Design review of the part built by this model. Coordinates are the model's own, in mm. A direction names the side the tool comes from. Coordinates: 2 decimals unless noted, no trailing zeros. Loops run counter-clockwise (first coordinate to the right, second up) from the corner with the lowest first, then second, coordinate; pieces in that order, holes last. Notation, with made-up numbers: (53.25, -16.75) - (89.25, -16.75) arc R7 ccw to (89.25, -12.75) - close; hole circle Ø5 at (61.25, 13). An arc over 180 degrees is marked (long way). Answer in a Markdown table with one row per item. Add a question column.
(1) Clearance check with flat-ended pins moving along their axes: pin 1 (1 mm diameter, centred on x = 10, y = 19.5, fed in from +Z); pin 2 (9 mm diameter, centred on y = 19.5, z = -10, fed in from -X); pin 3 (7.5 mm diameter, centred on x = 11, z = -7, fed in from +Y). State where each tip first meets the part, or that it passes through.
(2) We need section C-C, the plane y = 12.75. Write out the cut boundary in (x, z), plus the area to 3 significant figures.
(3) To check wall thickness, follow L1, parallel to X at y = 15, z = -11; L2, parallel to Y at x = 15, z = -1.5; L3, parallel to Z at x = 17.25, y = 13.25. State the ranges of each line that lie inside material, in increasing order. Write a range as [from, to].
(4) For faces 1 (the face through (20, 10, -16)), 2 (the face through (2.54, 11, -14)), list the 3-axis set-ups (+Z, -Z, +X, -X, +Y, -Y) from which the entire face can be reached by the end or side of a thin tool; tool diameter is ignored.
(5) The part is to be moulded in two halves that separate along X. For faces 3 (the face through (10, 6.35, -7)), 4 (the face through (12, 14, -19.05)), 5 (the face through (0, 9, -16)), 6 (the face through (10, 13, -25.4)), say which applies: released by +X, released by -X, zero draft, split by the parting line, or undercut.
(6) We need section B-B, the plane z = -20. Write out the cut boundary in (x, y) (3 decimals).
(7) We need section A-A, the plane y = 2. Write out the cut boundary in (x, z) (3 decimals).
(8) We need section D-D, the plane x = 10.25. Write out the cut boundary in (y, z), plus the area to 3 significant figures.
from build123d import *

# Parameters (mm, degrees)
BOSS_EXTRUDE1_DEPTH = 20
CUT_EXTRUDE1_DEPTH  = 20
CUT_EXTRUDE2_DEPTH  = 20
FILLET1_R           = 6.35
BOSS_EXTRUDE2_DEPTH = 19.05
CUT_EXTRUDE3_DEPTH  = 20.05
CUT_EXTRUDE4_DEPTH  = 21


with BuildPart() as part:
    # Sketch1 → Boss-Extrude1 (new body)
    with BuildSketch(Plane(origin=(0, 0, 0), x_dir=(0, 0, -1), z_dir=(1, 0, 0))):
        Polygon((0, 0), (0, 6.35), (19.05, 6.35), (19.05, 25.4), (25.4, 25.4), (25.4, 0), align=None)
    extrude(amount=BOSS_EXTRUDE1_DEPTH)

    # Sketch2 → Cut-Extrude1 (cut)
    with BuildSketch(Plane(origin=(0, 6.35, 0), x_dir=(1, 0, 0), z_dir=(0, 1, 0))):
        with BuildLine():
            ThreePointArc((8.37078656, 11.076825802), (7.750000055, 9.525), (8.37078656, 7.973174198))
            Line((8.37078656, 7.973174198), (10, 9.525))
            Line((10, 9.525), (8.37078656, 11.076825802))
        make_face()
        with BuildLine():
            Line((10, 9.525), (8.37078656, 7.973174198))
            ThreePointArc((8.37078656, 7.973174198), (10, 7.275000055), (11.62921344, 7.973174198))
            Line((11.62921344, 7.973174198), (10, 9.525))
        make_face()
        with BuildLine():
            Line((8.37078656, 11.076825802), (10, 9.525))
            Line((10, 9.525), (11.62921344, 11.076825802))
            ThreePointArc((11.62921344, 11.076825802), (10, 11.774999945), (8.37078656, 11.076825802))
        make_face()
        with BuildLine():
            Line((11.62921344, 11.076825802), (10, 9.525))
            Line((10, 9.525), (11.62921344, 7.973174198))
            ThreePointArc((11.62921344, 7.973174198), (12.089046422, 8.689305797), (12.249999945, 9.525))
            ThreePointArc((12.249999945, 9.525), (12.089046422, 10.360694203), (11.62921344, 11.076825802))
        make_face()
    extrude(amount=-CUT_EXTRUDE1_DEPTH, mode=Mode.SUBTRACT)

    # Sketch3 → Cut-Extrude2 (cut)
    with BuildSketch(Plane.XY.offset(-19.05)):
        with BuildLine():
            ThreePointArc((8.37078652, 17.42682584), (7.75, 15.875), (8.37078652, 14.32317416))
            Line((8.37078652, 14.32317416), (10, 15.875))
            Line((10, 15.875), (8.37078652, 17.42682584))
        make_face()
        with BuildLine():
            Line((10, 15.875), (8.37078652, 14.32317416))
            ThreePointArc((8.37078652, 14.32317416), (10, 13.625), (11.62921348, 14.32317416))
            Line((11.62921348, 14.32317416), (10, 15.875))
        make_face()
        with BuildLine():
            Line((8.37078652, 17.42682584), (10, 15.875))
            Line((10, 15.875), (11.62921348, 17.42682584))
            ThreePointArc((11.62921348, 17.42682584), (10, 18.125), (8.37078652, 17.42682584))
        make_face()
        with BuildLine():
            Line((11.62921348, 17.42682584), (10, 15.875))
            Line((10, 15.875), (11.62921348, 14.32317416))
            ThreePointArc((11.62921348, 14.32317416), (12.089046473, 15.039305777), (12.25, 15.875))
            ThreePointArc((12.25, 15.875), (12.089046473, 16.710694223), (11.62921348, 17.42682584))
        make_face()
    extrude(amount=-CUT_EXTRUDE2_DEPTH, mode=Mode.SUBTRACT)

    # Fillet1
    fillet1_edges = [part.edges().sort_by_distance(p)[0] for p in [
        (20, 25.4, -22.225),
        (20, 3.175, 0),
        (0, 3.175, 0),
        (0, 25.4, -22.225),
    ]]
    fillet(fillet1_edges, radius=FILLET1_R)

    # Sketch4 → Boss-Extrude2 (add)
    with BuildSketch(Plane(origin=(0, 6.35, 0), x_dir=(1, 0, 0), z_dir=(0, 1, 0))):
        with BuildLine():
            Line((2.54, 1.27), (2.54, 19.05))
            Line((2.54, 19.05), (0, 19.05))
            Line((0, 19.05), (0, 6.35))
            ThreePointArc((0, 6.35), (0.670387337, 3.510193669), (2.54, 1.27))
        make_face()
        with BuildLine():
            Line((20, 19.05), (17.46, 19.05))
            Line((17.46, 19.05), (17.46, 1.27))
            ThreePointArc((17.46, 1.27), (19.329612663, 3.510193669), (20, 6.35))
            Line((20, 6.35), (20, 19.05))
        make_face()
    extrude(amount=BOSS_EXTRUDE2_DEPTH)

    # Sketch5 → Cut-Extrude3 (cut, through all)
    with BuildSketch(Plane(origin=(0, 0, -19.05), x_dir=(-1, 0, 0), z_dir=(0, 0, -1))):
        with BuildLine():
            Line((0, 19.05), (0, 25.4))
            Line((0, 25.4), (-2.54, 25.4))
            Line((-2.54, 25.4), (-2.54, 24.13))
            ThreePointArc((-2.54, 24.13), (-0.670387337, 21.889806331), (0, 19.05))
        make_face()
        with BuildLine():
            Line((-17.46, 24.13), (-17.46, 25.4))
            Line((-17.46, 25.4), (-20, 25.4))
            Line((-20, 25.4), (-20, 19.05))
            ThreePointArc((-20, 19.05), (-19.329612663, 21.889806331), (-17.46, 24.13))
        make_face()
    extrude(amount=-CUT_EXTRUDE3_DEPTH, mode=Mode.SUBTRACT)

    # Sketch6 → Cut-Extrude4 (cut, through all)
    with BuildSketch(Plane.ZY):
        Polygon((-13.97, 19.05), (-6.35, 19.05), (-6.35, 11.43), (-1.27, 6.35), (-1.27, 24.13), (-19.05, 24.13), align=None)
        Polygon((-6.35, 11.43), (-6.35, 19.05), (-13.97, 19.05), align=None)
    extrude(amount=-CUT_EXTRUDE4_DEPTH, mode=Mode.SUBTRACT)


solid = part.part
Responses:
| question | item | result |
|---|---|---|
| 1 | pin 1 | stops at z = -19.05 |
| 1 | pin 2 | stops at x = 0 |
| 1 | pin 3 | stops at y = 6.35 |
| 2 | outline | (0, -25.4) - (20, -25.4) - (20, -7.67) - (17.46, -7.67) - (17.46, -19.05) - (2.54, -19.05) - (2.54, -7.67) - (0, -7.67) - close |
| 2 | area | 185 mm2 |
| 3 | L1 | x = [0, 2.54], [17.46, 20] |
| 3 | L2 | y = [0, 6.35] |
| 3 | L3 | z = [-25.4, -19.05] |
| 4 | face 1 | +Z, -Z, +X, +Y, -Y |
| 4 | face 2 | +Z, +Y |
| 5 | face 3 | undercut |
| 5 | face 4 | undercut |
| 5 | face 5 | released by -X |
| 5 | face 6 | zero draft |
| 6 | outline | (0, 0) - (20, 0) - (20, 19.05) arc R6.35 ccw to (13.65, 25.4) - (6.35, 25.4) arc R6.35 ccw to (0, 19.05) - close; hole circle Ø4.5 at (10, 15.875) |
| 7 | outline | (0, -25.4) - (20, -25.4) - (20, -6.35) arc R6.35 ccw to (13.65, 0) - (6.35, 0) arc R6.35 ccw to (0, -6.35) - close; hole circle Ø4.5 at (10, -9.525) |
| 8 | outline | (0, -25.4) - (13.64, -25.4) - (13.64, -19.05) - (6.35, -19.05) - (6.35, -11.76) - (0, -11.76) - close; (0, -7.29) - (6.35, -7.29) - (6.35, 0) - (0, 0) - close; (18.11, -25.4) - (25.4, -25.4) - (25.4, -19.05) - (18.11, -19.05) - close |
| 8 | area | 225 mm2 |
